Part print with two shaded views. Sizes in mm from the minimum x, y, z corner. A direction names the side the tool comes from. Coordinates: 2 decimals unless noted, no trailing zeros. Write each loop counter-clockwise with the first axis right and the second up, starting at its lowest first coordinate (ties: lowest second). Pieces come first, ordered by that corner, then holes. Notation, with made-up numbers: (6.25, 54.5) - (50.25, 54.5) arc R16 cw to (50.25, 61.5) - close; hole circle Ø10 at (82.5, 21.5). An arc over 180 degrees is marked (long way). Answer in a Markdown table with one row per item. Add a question column.
Q1. Two-plate mould, pull along X, no slides. Class the marked faces 1, 2 and 3: +X half, -X half, draft (parallel to the pull), parting line (faces both ways), or undercut.
Q2. Pin check, flat tips, straight feed: pin 1 (10 mm diameter, centred on x = 3.5, z = 17.5, fed in from -Y); pin 2 (0.9 mm diameter, centred on x = 9.5, y = 5.5, fed in from +Z); pin 3 (1.5 mm diameter, centred on x = 9.5, y = 6, fed in from -Z). Stop position of each tip, or through.
Q3. Band-saw the part on C-C (x = 9.5). List the corners of the cut face in (y, z), and give its area (3 significant figures).
Q4. Drill centre lines: line 1 along Y through (x, z) = (9.5, 2.95); line 2 along Z through (x, y) = (15.25, 15.75); line 3 along Y through (x, z) = (5.5, 2.9). Where is each one in solid material? Low to high. Write a range as from..to.
Q5. Band-saw the part on A-A (y = 9.5). List the corners of the cut face in (x, z).
Q6. Band-saw the part on B-B (z = 2.25). List the corners of the cut face in (x, y), and give its area (3 significant figures).
Q7. 3-axis set-ups, long thin cutter, end or side, ignore diameter. For the marked faces 4 and 5: which of +Z, -Z, +X, -X, +Y, -Y reach the whole face in a straight line?
Q8. Band-saw the part on D-D (z = 20.5). List the corners of the cut face in (x, y).
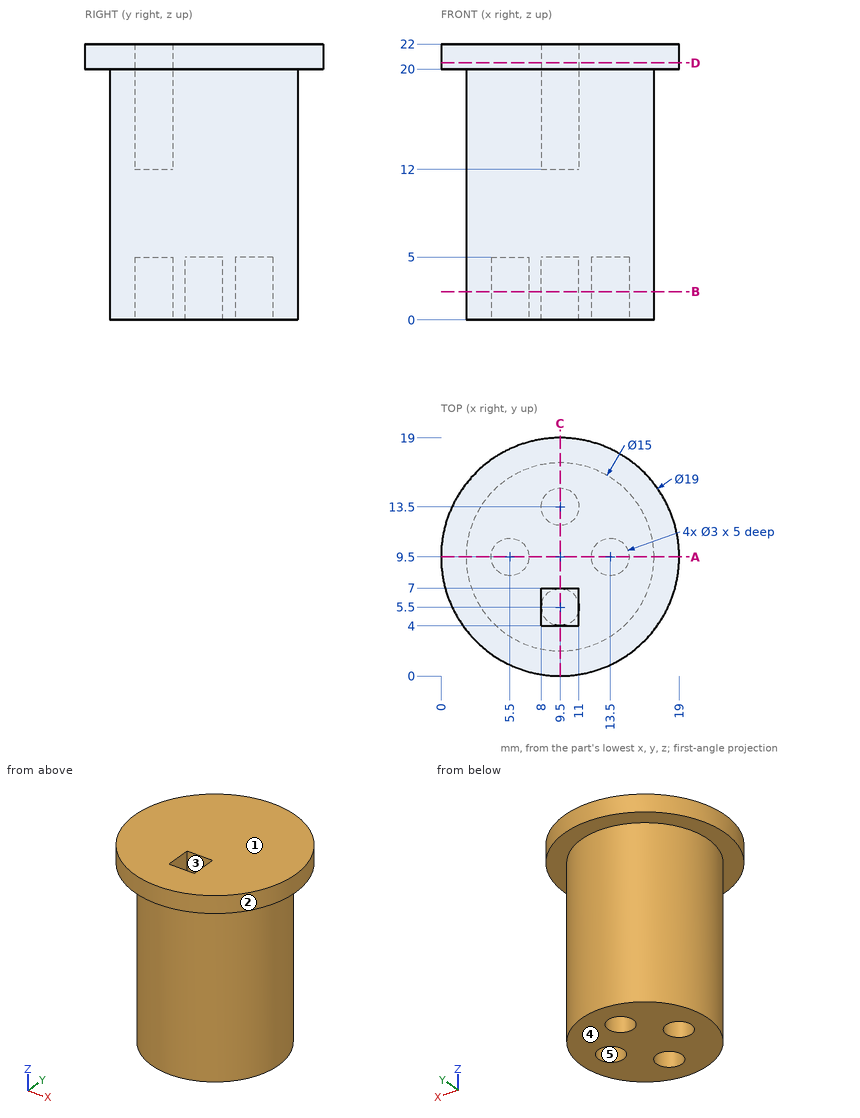
Checked values:
| question | item | result |
|---|---|---|
| 1 | face 1 | draft |
| 1 | face 2 | parting line |
| 1 | face 3 | undercut |
| 2 | pin 1 | stops at y = 0.15 |
| 2 | pin 2 | stops at z = 12 |
| 2 | pin 3 | stops at z = 5 |
| 3 | outline | (0, 20) - (2, 20) - (2, 0) - (4, 0) - (4, 5) - (7, 5) - (7, 0) - (12, 0) - (12, 5) - (15, 5) - (15, 0) - (17, 0) - (17, 20) - (19, 20) - (19, 22) - (7, 22) - (7, 12) - (4, 12) - (4, 22) - (0, 22) - close |
| 3 | area | 278 mm² |
| 4 | line 1 | y = 2..4, 7..12, 15..17 |
| 4 | line 2 | z = 20..22 |
| 4 | line 3 | y = 3.16..8, 11..15.84 |
| 5 | outline | (0, 20) - (2, 20) - (2, 0) - (4, 0) - (4, 5) - (7, 5) - (7, 0) - (12, 0) - (12, 5) - (15, 5) - (15, 0) - (17, 0) - (17, 20) - (19, 20) - (19, 22) - (0, 22) - close |
| 6 | outline | circle Ø15 at (9.5, 9.5); hole circle Ø3 at (5.5, 9.5); hole circle Ø3 at (9.5, 5.5); hole circle Ø3 at (9.5, 13.5); hole circle Ø3 at (13.5, 9.5) |
| 6 | area | 148 mm² |
| 7 | face 4 | -Z, +X, -X, +Y, -Y |
| 7 | face 5 | -Z |
| 8 | outline | circle Ø19 at (9.5, 9.5); hole (8, 4) - (11, 4) - (11, 7) - (8, 7) - close |
